Design review of the part built by this model. Coordinates are the model's own, in mm. A direction names the side the tool comes from. Coordinates: 2 decimals unless noted, no trailing zeros. Loops run counter-clockwise (first coordinate to the right, second up) from the corner with the lowest first, then second, coordinate; pieces in that order, holes last. Notation, with made-up numbers: (-20, 66) - (19, 66) arc R30 ccw to (19, 96) - close; hole circle Ø6 at (81, -29). An arc over 180 degrees is marked (long way). Answer in a Markdown table with one row per item. Add a question column.
(1) The part is to be moulded in two halves that separate along X. For faces 3 (the face through (-7.4, -12.1, 0)), 4 (the face through (13.04, -5.41, 43.88)), 5 (the face through (-1.63, -7.32, 48.99)), say which applies: released by +X, released by -X, zero draft, split by the parting line, or undercut.
(2) For faces 1 (the face through (-6, -5, 50)), 2 (the face through (12.932, -5.362, 45.972)), list the 3-axis set-ups (+Z, -Z, +X, -X, +Y, -Y) from which the entire face can be reached by the end or side of a thin tool; tool diameter is ignored.
(3) Clearance check with flat-ended pins moving along their axes: pin 1 (2 mm diameter, centred on y = 10, z = 11.5, fed in from -X); pin 2 (10 mm diameter, centred on x = -11.5, z = 13.5, fed in from -Y); pin 3 (4 mm diameter, centred on x = -11, z = 39.5, fed in from -Y). State where each tip first meets the part, or that it passes through.
(4) We need section A-A, the plane z = 4.5. Write out the cut boundary in (x, y), plus the area to 3 significant figures.
(5) To check wall thickness, follow L1, parallel to Y at x = 0, z = 36.05; L2, parallel to X at y = -13, z = 4; L3, parallel to Y at x = -4, z = 33.5. State the ranges of each line that lie inside material, in increasing order. Write a range as [from, to].
from build123d import *

# Parameters (mm, degrees)
F0_R          = 16.5
F0_R_2        = 14
F1_DEPTH      = 40
F2_R          = 14
F2_R_2        = 7.5
F3_DEPTH      = 10
F3_DEPTH_BACK = 5
F4_S5_R       = 16.5
F4_T6_DEPTH   = 27
F5_SIZE       = 2
F6_S5_R       = 14
F6_T6_DEPTH   = 24
F7_SIZE       = 5


# Not quite as in the source:
# - a fillet or chamfer that OpenCascade refuses, or shapes differently, is made with other operations: its cross-section is extruded or revolved along the edge and cut away or added


with BuildPart() as f1:
    # F0 (on Top) → F1 (new body)
    with BuildSketch(Plane.XY):
        Circle(F0_R)
        Circle(F0_R_2, mode=Mode.SUBTRACT)
    extrude(amount=F1_DEPTH)

    # F2 (on face) → F3 (join, two sides)
    with BuildSketch(Plane.XY.offset(40)) as f3_sk:
        Circle(F2_R)
        Circle(F2_R_2, mode=Mode.SUBTRACT)
    extrude(amount=F3_DEPTH)
    extrude(f3_sk.sketch, amount=-F3_DEPTH_BACK)

    # F4: chamfer of 4 on 1 edges, made by hand


with BuildPart() as f4_tool2:
    # F4_s3 → F4_t4 (revolve)
    with BuildSketch(Plane.XZ):
        Polygon((18, 40), (14, 44), (14, 40), align=None)
    revolve(axis=Axis((0, 0, 40), (0, 0, 1)))

    # F4_s5 → F4_t6 (intersect, symmetric)
    with BuildSketch(Plane.XY.offset(42)):
        Circle(F4_S5_R)
    extrude(amount=F4_T6_DEPTH, both=True, mode=Mode.INTERSECT)


with BuildPart() as f1_1:
    add(f1.part)

    # F4_t1: union F4_tool2
    add(f4_tool2.part)

    # F5
    f5_edges = [f1_1.edges().sort_by_distance(p)[0] for p in [
        (-14, 0, 50),
    ]]
    chamfer(f5_edges, length=F5_SIZE)

    # F6: chamfer of 8 on 1 edges, made by hand


with BuildPart() as f6_tool2:
    # F6_s3 → F6_t4 (revolve)
    with BuildSketch(Plane.XZ):
        Polygon((7.5, 43), (15.5, 35), (7.5, 35), align=None)
    revolve(axis=Axis((0, 0, 35), (0, 0, 1)))

    # F6_s5 → F6_t6 (intersect, symmetric)
    with BuildSketch(Plane.XY.offset(39)):
        Circle(F6_S5_R)
    extrude(amount=F6_T6_DEPTH, both=True, mode=Mode.INTERSECT)


with BuildPart() as f1_2:
    add(f1_1.part)

    # F6_t1: cut F6_tool2
    add(f6_tool2.part, mode=Mode.SUBTRACT)

    # F7
    f7_edges = [f1_2.edges().sort_by_distance(p)[0] for p in [
        (-7.5, 0, 43),
    ]]
    chamfer(f7_edges, length=F7_SIZE)


solid = f1_2.part
Responses:
| question | item | result |
|---|---|---|
| 1 | face 3 | zero draft |
| 1 | face 4 | split by the parting line |
| 1 | face 5 | undercut |
| 2 | face 1 | +Z, +X, -X, +Y, -Y |
| 2 | face 2 | +Z |
| 3 | pin 1 | stops at x = -13.83 |
| 3 | pin 2 | stops at y = -15.17 |
| 3 | pin 3 | stops at y = -13.83 |
| 4 | outline | circle Ø33 at (0, 0); hole circle Ø28 at (0, 0) |
| 4 | area | 240 mm2 |
| 5 | L1 | y = [-16.5, -14], [14, 16.5] |
| 5 | L2 | x = [-10.16, -5.2], [5.2, 10.16] |
| 5 | L3 | y = [-16.01, -13.42], [13.42, 16.01] |
